Could you check a few things on this model? Use its own coordinates, in mm. Round coordinates to 2 decimals unless told otherwise and drop trailing zeros. Order: outer loops, then holes, each group sorted by start corner. A loop starts at its lowest first (then second) coordinate and runs counter-clockwise, first axis right, second up. Notation, with made-up numbers: (83.25, 73.25) -> (126.25, 73.25) arc R16 ccw to (126.25, 83.25) -> close; hole circle Ø10 at (14, 68.5). An arc over 180 degrees is marked (long way). One line per question, with ' | ' between items.
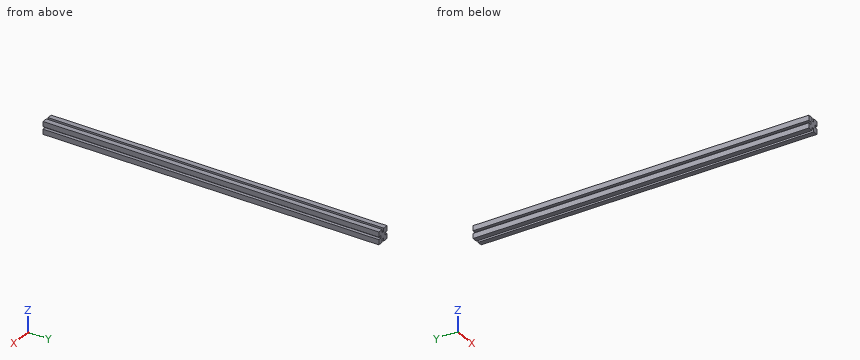
```python
from build123d import *

# Parameters (mm, degrees)
BOSS_EXTRUDE1_DEPTH = 1338
BOSS_EXTRUDE2_DEPTH = 10


with BuildPart() as part:
    # Sketch1 → Boss-Extrude1 (new body)
    with BuildSketch(Plane(origin=(0, 0, 0), x_dir=(1, 0, 0), z_dir=(0, 1, 0))):
        Polygon((-25, 25), (-5, 25), (-5, 12.5), (5, 12.5), (5, 25), (25, 25), (25, 5), (12.5, 5), (12.5, -5), (25, -5), (25, -25), (5, -25), (5, -12.5), (-5, -12.5), (-5, -25), (-25, -25), (-25, -5), (-12.5, -5), (-12.5, 5), (-25, 5), align=None)
    extrude(amount=BOSS_EXTRUDE1_DEPTH)

    # Sketch1<2> → Boss-Extrude2 (add)
    with BuildSketch(Plane(origin=(0, 0, 0), x_dir=(1, 0, 0), z_dir=(0, 1, 0))):
        Polygon((-25, 25), (-5, 25), (-5, 12.5), (5, 12.5), (5, 25), (25, 25), (25, 5), (12.5, 5), (12.5, -5), (25, -5), (25, -25), (5, -25), (5, -12.5), (-5, -12.5), (-5, -25), (-25, -25), (-25, -5), (-12.5, -5), (-12.5, 5), (-25, 5), align=None)
    extrude(amount=BOSS_EXTRUDE2_DEPTH)


solid = part.part
```
1. I'm going to push a flat-ended pin straight in: pin 1 (3 mm diameter, centred on x = -1, y = 632.5, fed in from +Z). Where does the tip first touch, or does it pass through?
From the geometry:
pin 1: stops at z = 12.5
2. I want a section at A-A on y = 1118.5. List the corners of the cut face in (x, z) for me.
From the geometry:
outline: (-25, -25) -> (-5, -25) -> (-5, -12.5) -> (5, -12.5) -> (5, -25) -> (25, -25) -> (25, -5) -> (12.5, -5) -> (12.5, 5) -> (25, 5) -> (25, 25) -> (5, 25) -> (5, 12.5) -> (-5, 12.5) -> (-5, 25) -> (-25, 25) -> (-25, 5) -> (-12.5, 5) -> (-12.5, -5) -> (-25, -5) -> close
3. I need wall thicknesses on probe 1 along Z at (x, y) = (-19, 1274); probe 2 along Z at (x, y) = (-2, 131). Which ranges of each line are inside material? Lowest first, please.
From the geometry:
probe 1: z = -25 to -5, 5 to 25 | probe 2: z = -12.5 to 12.5
